```python
from build123d import *

# Parameters (mm, degrees)
SKETCH_1_R          = 1.25
EXTRUDE_1_DEPTH     = 12
SKETCH_3_R          = 1.25
CUT_EXTRUDE_1_DEPTH = 8.5
FILLET_1_R          = 10


with BuildPart() as part:
    # ｽｹｯﾁ1 → ﾎﾞｽ - 押し出し1 (new body)
    with BuildSketch(Plane.XY):
        with BuildLine():
            Line((-9.797958971, 10), (9.797958971, 10))
            ThreePointArc((9.797958971, 10), (0, -14), (-9.797958971, 10))
        make_face()
        with Locations((-8.660254038, 5)):
            Circle(SKETCH_1_R, mode=Mode.SUBTRACT)
        with Locations((8.660254038, 5)):
            Circle(SKETCH_1_R, mode=Mode.SUBTRACT)
        with Locations((0, -10)):
            Circle(SKETCH_1_R, mode=Mode.SUBTRACT)
        with BuildLine():
            Line((-1.322875656, 1.5), (1.322875656, 1.5))
            ThreePointArc((1.322875656, 1.5), (0, -2), (-1.322875656, 1.5))
        make_face(mode=Mode.SUBTRACT)
    extrude(amount=EXTRUDE_1_DEPTH)

    # ｽｹｯﾁ3 → ｶｯﾄ - 押し出し1 (cut)
    with BuildSketch(Plane(origin=(0, 10, 0), x_dir=(1, 0, 0), z_dir=(0, 1, 0))):
        with Locations(Location((0, -8, 0), (0, 0, 270))):
            Circle(SKETCH_3_R)
    extrude(amount=-CUT_EXTRUDE_1_DEPTH, mode=Mode.SUBTRACT)

    # ﾌｨﾚｯﾄ1
    fillet_1_edges = [part.edges().sort_by_distance(p)[0] for p in [
        (-9.797958971, 10, 6),
        (9.797958971, 10, 6),
    ]]
    fillet(fillet_1_edges, radius=FILLET_1_R)


solid = part.part
```
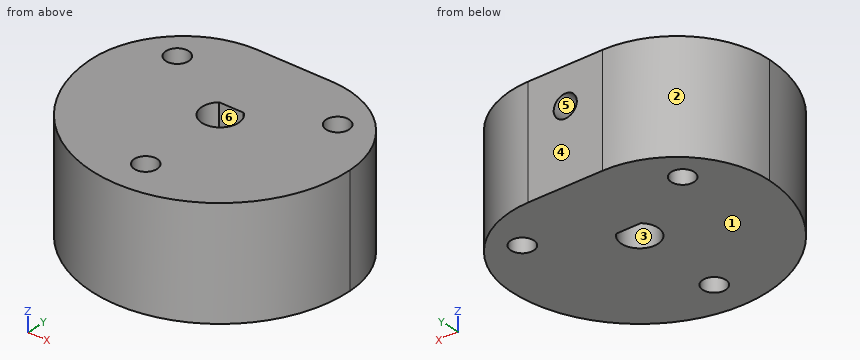
Geometry check sheet. Reference: the model listing, model coordinates, mm. Face numbers are marked on the shaded views. A direction names the side the tool comes from. Give positions to 0.01 mm unless a question says otherwise; leave off trailing zeros. Write each loop counter-clockwise with the first axis right and the second up, starting at its lowest first coordinate (ties: lowest second). Pieces come first, ordered by that corner, then holes. Notation, with made-up numbers: (59, 7) -> (95, 7) arc R17 ccw to (95, 25) -> close; hole circle Ø3 at (-30.5, -11.75). An arc over 180 degrees is marked (long way). Use one line per item in the form item = value.
Item 1: Sectioned sample at B-B on x = 0. Enter the section's corners in (y, z).
Results list:
outline = (-14, 0) -> (-11.25, 0) -> (-11.25, 12) -> (-14, 12) -> close; (-8.75, 0) -> (-2, 0) -> (-2, 12) -> (-8.75, 12) -> close; (1.5, 0) -> (10, 0) -> (10, 6.75) -> (1.5, 6.75) -> close; (1.5, 9.25) -> (10, 9.25) -> (10, 12) -> (1.5, 12) -> close
Item 2: Depth check by flat-ended pin: pin 1 Ø6 at (y, z) = (-6, 10) entering from +X; pin 2 Ø2 at (x, y) = (0, -10) entering from +Z; pin 3 Ø2 at (y, z) = (-10.5, 1.5) entering from +X; pin 4 Ø2 at (x, z) = (9, 4) entering from -Y. Enter the tip coordinate at first touch or a pass-through.
Results list:
pin_1 = 13.67
pin_2 = through
pin_3 = 10.28
pin_4 = -11.49
Item 3: Scan lines: line 1 (X direction, y = 4, z = 7.75); line 2 (Y direction, x = 9.5, z = 2.75); line 3 (X direction, y = 8, z = 8). Record each from-to range of solid material in increasing order.
Results list:
line_1 = -13.17 to -9.41, -7.91 to -1.22, 1.22 to 7.91, 9.41 to 13.17
line_2 = -10.28 to 4.07, 5.93 to 8.35
line_3 = -10 to -1.25, 1.25 to 10
Item 4: Access from +Z, -Z, +X, -X, +Y, -Y to the whole of each face (thin tool, end or side, straight path). Record for the marked faces 4, 5 and 6.
Results list:
face_4 = +Z, -Z, +X, -X, +Y
face_5 = +Y
face_6 = +Z, -Z
Item 5: Mould release check, pull along Y, two halves, no side actions. Record for the marked faces 1, 2 and 3: released by +Y, released by -Y, zero draft, split by the parting line, or undercut.
Results list:
face_1 = zero draft
face_2 = released by +Y
face_3 = undercut
Item 6: Sectioned sample at A-A on y = 5. Enter the section's corners in (x, z).
Results list:
outline = (-12.66, 0) -> (-9.91, 0) -> (-9.91, 12) -> (-12.66, 12) -> close; (-7.41, 0) -> (7.41, 0) -> (7.41, 12) -> (-7.41, 12) -> close; (9.91, 0) -> (12.66, 0) -> (12.66, 12) -> (9.91, 12) -> close; hole circle Ø2.5 at (0, 8)
Item 7: Sectioned sample at C-C on z = 2.5. Enter the section's corners in (x, y), plus the area to 3 significant figures.
Results list:
outline = (-14, 0) arc R14 ccw to (14, 0) arc R10 ccw to (4, 10) -> (-4, 10) arc R10 ccw to start; hole circle Ø2.5 at (-8.66, 5); hole (-1.32, 1.5) arc R2 ccw (long way) to (1.32, 1.5) -> close; hole circle Ø2.5 at (0, -10); hole circle Ø2.5 at (8.66, 5)
area = 519 mm2
Item 8: Sectioned sample at D-D on z = 7.5. Enter the section's corners in (x, y), plus the area to 3 significant figures.
Results list:
outline = (-14, 0) arc R14 ccw to (14, 0) arc R10 ccw to (4, 10) -> (1.15, 10) -> (1.15, 1.5) -> (1.32, 1.5) arc R2 cw (long way) to (-1.32, 1.5) -> (-1.15, 1.5) -> (-1.15, 10) -> (-4, 10) arc R10 ccw to start; hole circle Ø2.5 at (-8.66, 5); hole circle Ø2.5 at (0, -10); hole circle Ø2.5 at (8.66, 5)
area = 499 mm2
